from build123d import *

# Parameters (mm, degrees)
SKETCH1_R           = 1.7
BOSS_EXTRUDE1_DEPTH = 5


with BuildPart() as part:
    # Sketch1 → Boss-Extrude1 (new body)
    with BuildSketch(Plane.XY):
        with BuildLine():
            ThreePointArc((-37.834642703, 12.842889611), (-38.606977712, 11.916261554), (-39.134911245, 10.831629309))
            Line((-39.134911245, 10.831629309), (-39.354944681, 10.193532345))
            ThreePointArc((-39.354944681, 10.193532345), (-39.123029117, 6.373731812), (-36.25803319, 3.83671402))
            Line((-36.25803319, 3.83671402), (-29.668188839, 1.564353899))
            ThreePointArc((-29.668188839, 1.564353899), (-26.491164954, 1.536581811), (-23.938801839, 3.428589895))
            Line((-23.938801839, 3.428589895), (-23.309086795, 4.330374611))
            ThreePointArc((-23.309086795, 4.330374611), (-21.521238753, 5.901319007), (-19.20965321, 6.467745699))
            Line((-19.20965321, 6.467745699), (-17.817780351, 6.467745699))
            ThreePointArc((-17.817780351, 6.467745699), (-15.427188658, 5.859222826), (-13.618488855, 4.181774242))
            Line((-13.618488855, 4.181774242), (-10.381594688, -0.826523177))
            ThreePointArc((-10.381594688, -0.826523177), (-7.83372555, -2.83190182), (-4.59138835, -2.852641252))
            Line((-4.59138835, -2.852641252), (4.902899214, 0.333885288))
            Line((4.902899214, 0.333885288), (17.263606315, 5.252218218))
            ThreePointArc((17.263606315, 5.252218218), (19.830876998, 7.552622541), (20.299269541, 10.967786846))
            Line((20.299269541, 10.967786846), (18.310232366, 20.048547406))
            ThreePointArc((18.310232366, 20.048547406), (18.19566052, 20.478915648), (18.043247633, 20.897381709))
            Line((18.043247633, 20.897381709), (12.643097146, 33.892720517))
            Line((12.643097146, 33.892720517), (7.177182545, 44.720280021))
            ThreePointArc((7.177182545, 44.720280021), (6.821120261, 45.642450212), (6.653441068, 46.616648291))
            Line((6.653441068, 46.616648291), (5.174876069, 67.279164767))
            ThreePointArc((5.174876069, 67.279164767), (4.105623253, 70.028623013), (1.672465938, 71.696726041))
            Line((1.672465938, 71.696726041), (0.300566202, 72.123383215))
            ThreePointArc((0.300566202, 72.123383215), (-0.512819916, 72.303655469), (-1.344848079, 72.346366128))
            Line((-1.344848079, 72.346366128), (-13.585713544, 71.953043516))
            ThreePointArc((-13.585713544, 71.953043516), (-16.669785637, 70.75986422), (-18.33462528, 67.902682661))
            ThreePointArc((-18.33462528, 67.902682661), (-17.88389808, 65.164771828), (-16.042829318, 63.088771694))
            Line((-16.042829318, 63.088771694), (-11.247293049, 60.054506954))
            ThreePointArc((-11.247293049, 60.054506954), (-9.367982736, 57.896266905), (-8.980115504, 55.060889264))
            Line((-8.980115504, 55.060889264), (-10.526035755, 45.120570864))
            Line((-10.526035755, 45.120570864), (-33.479905595, 16.940953472))
            Line((-33.479905595, 16.940953472), (-37.834642703, 12.842889611))
        make_face()
        with Locations((-31.17879703, 9.476441992)):
            Circle(SKETCH1_R, mode=Mode.SUBTRACT)
        with Locations((-6.681396598, 4.488719859)):
            Circle(SKETCH1_R, mode=Mode.SUBTRACT)
        with Locations((13.146755278, 7.104898975)):
            Circle(SKETCH1_R, mode=Mode.SUBTRACT)
    extrude(amount=BOSS_EXTRUDE1_DEPTH)


solid = part.part
Work out the finished part from the listing and answer in its coordinate system (mm). A direction names the side the tool comes from. Round coordinates to 2 decimals unless told otherwise and drop trailing zeros. Write each loop counter-clockwise with the first axis right and the second up, starting at its lowest first coordinate (ties: lowest second). Pieces come first, ordered by that corner, then holes. Notation, with made-up numbers: (-2, 34.5) -> (25, 34.5) arc R24 cw to (25, 53.5) -> close; hole circle Ø11 at (39, -14). An arc over 180 degrees is marked (long way). Answer as CSV lines item,"result". Start each with the question number.
(1) Find the intervals of material crossed by probe 1 along Y at (x, z) = (-16.5, 2.7); probe 2 along Y at (x, z) = (-6, 3.2); probe 3 along X at (y, z) = (46, 4.55), in increasing order.
(2) The part is cut by section B-B, the plane x = 3. Give the vertices of the cut face in (y, z).
(3) The part is cut by section C-C, the plane y = 61. Give the vertices of the cut face in (x, z), then the cut area to 3 significant figures.
(4) The mould has two halves that part along X. Classify faces 4 (the flat face through (15.381, 27.304, 2.465)), 5 (the flat face through (-9.742, 50.16, 2.465)), 6 (the cylindrical face through (14.717, 6.454, 2.465)): +X half, -X half, draft (parallel to the pull), parting line (faces both ways), or undercut.
(5) A tool of negligible diameter and unlimited length cuts with its end or side. For faces 1 (the flat face through (9.95, 39.23, 2.46)), 2 (the flat face through (-13.679, 61.593, 2.465)), 3 (the flat face through (-12.02, 1.71, 2.46)), from which of +Z, -Z, +X, -X, +Y, -Y can it reach the whole face along a straight path? Write none if from no direction.
(6) Each of these flat-tipped pins is pushed along its axis until it touches: pin 1 (0.7 mm diameter, centred on x = -18.5, z = 2, fed in from -Y); pin 2 (3 mm diameter, centred on x = 2.5, z = 2, fed in from +Y). Where does it stop, or does it pass through?
(7) The part is cut by section A-A, the plane z = 3.5. Give the number of separate pieces and of enclosed holes in the cut face, then the cut area to 3 significant figures.
Output values:
1,probe 1,"y = 6.29 to 37.79, 63.42 to 70.9"
1,probe 2,"y = -3.11 to 2.93, 6.05 to 72.2"
1,probe 3,"x = -10.39 to 6.74"
2,outline,"(-0.3, 0) -> (71.06, 0) -> (71.06, 5) -> (-0.3, 5) -> close"
3,outline,"(-12.74, 0) -> (5.62, 0) -> (5.62, 5) -> (-12.74, 5) -> close"
3,area,"91.8 mm²"
4,face 4,"+X half"
4,face 5,"-X half"
4,face 6,"undercut"
5,face 1,"+Z, -Z, +X, +Y"
5,face 2,"+Z, -Z, -X"
5,face 3,"+Z, -Z, -Y"
6,pin 1,"stops at y = 6.47"
6,pin 2,"stops at y = 71.91"
7,separate pieces,"1"
7,enclosed holes,"3"
7,area,"2,330 mm²"
